Design review of the part built by this model. Coordinates are the model's own, in mm. A direction names the side the tool comes from. Coordinates: 2 decimals unless noted, no trailing zeros. Loops run counter-clockwise (first coordinate to the right, second up) from the corner with the lowest first, then second, coordinate; pieces in that order, holes last. Notation, with made-up numbers: (-39, 26) -> (-9, 26) arc R30 ccw to (-9, 52) -> close; hole circle Ø10 at (-24.5, -27). An arc over 180 degrees is marked (long way). Answer in a Markdown table with one row per item.
```python
from build123d import *

# Parameters (mm, degrees)
SKETCH3_R           = 2.4
BOSS_EXTRUDE1_DEPTH = 20
BOSS_EXTRUDE2_START = -15
SKETCH3_4_W         = 6.6
SKETCH3_4_H         = 6.6
SKETCH3_4_R         = 2.4
BOSS_EXTRUDE2_DEPTH = 15
BOSS_EXTRUDE3_DEPTH = 2


with BuildPart() as part:
    # Sketch3 → Boss-Extrude1 (new body)
    with BuildSketch(Plane.XY):
        Circle(SKETCH3_R)
    extrude(amount=BOSS_EXTRUDE1_DEPTH)

    # Sketch3_4 → Boss-Extrude2 (add)
    # profile 1 of 2: a face of its own
    with BuildSketch(Plane.XY.offset(BOSS_EXTRUDE2_START)):
        Rectangle(SKETCH3_4_W, SKETCH3_4_H)
        Circle(SKETCH3_4_R, mode=Mode.SUBTRACT)
    # profile 2 of 2: a face of its own
    with BuildSketch(Plane.XY.offset(BOSS_EXTRUDE2_START)):
        Circle(SKETCH3_4_R)
    extrude(amount=BOSS_EXTRUDE2_DEPTH)

    # Sketch3_5 → Boss-Extrude3 (add)
    with BuildSketch(Plane.XY):
        Polygon((3.3, 3.3), (3.3, -3.3), (5.3, -3.3), (5.3, 5.3), (-5.3, 5.3), (-5.3, -3.3), (-3.3, -3.3), (-3.3, 3.3), align=None)
    extrude(amount=-BOSS_EXTRUDE3_DEPTH)


solid = part.part
```
(1) To check wall thickness, follow probe 1 along X at (y, z) = (1, -13); probe 2 along Z at (x, y) = (2, 3); probe 3 along Z at (x, y) = (4.25, 4). State the ranges of each line that lie inside material, in increasing order.
Evaluation:
| item | result |
|---|---|
| probe 1 | x = -3.3 to 3.3 |
| probe 2 | z = -15 to 0 |
| probe 3 | z = -2 to 0 |
(2) Take a section at A-A on x = 0. Give the boundary of the cut face in (y, z), and give its area (3 significant figures).
Evaluation:
| item | result |
|---|---|
| outline | (-3.3, -15) -> (3.3, -15) -> (3.3, -2) -> (5.3, -2) -> (5.3, 0) -> (2.4, 0) -> (2.4, 20) -> (-2.4, 20) -> (-2.4, 0) -> (-3.3, 0) -> close |
| area | 199 mm² |
(3) For pin 1 (2 mm diameter, centred on x = 3.5, z = 2, fed in from +Y); pin 2 (2 mm diameter, centred on y = -1.5, z = -9, fed in from +X); pin 3 (3 mm diameter, centred on y = -2, z = 2, fed in from -X); pin 4 (5.5 mm diameter, centred on x = 1, z = -9.5, fed in from +Y), all flat-tipped, find the tip position at first contact; note any pin that passes through.
Evaluation:
| item | result |
|---|---|
| pin 1 | passes through |
| pin 2 | stops at x = 3.3 |
| pin 3 | stops at x = -2.35 |
| pin 4 | stops at y = 3.3 |
(4) Take a section at C-C on z = -11.5. Give the boundary of the cut face in (x, y), and give its area (3 significant figures).
Evaluation:
| item | result |
|---|---|
| outline | (-3.3, -3.3) -> (3.3, -3.3) -> (3.3, 3.3) -> (-3.3, 3.3) -> close |
| area | 43.6 mm² |
(5) Take a section at D-D on y = -1.5. Give the boundary of the cut face in (x, z), and give its area (3 significant figures).
Evaluation:
| item | result |
|---|---|
| outline | (-5.3, -2) -> (-3.3, -2) -> (-3.3, -15) -> (3.3, -15) -> (3.3, -2) -> (5.3, -2) -> (5.3, 0) -> (1.87, 0) -> (1.87, 20) -> (-1.87, 20) -> (-1.87, 0) -> (-5.3, 0) -> close |
| area | 182 mm² |
(6) Take a section at B-B on y = 0. Give the boundary of the cut face in (x, z).
Evaluation:
| item | result |
|---|---|
| outline | (-5.3, -2) -> (-3.3, -2) -> (-3.3, -15) -> (3.3, -15) -> (3.3, -2) -> (5.3, -2) -> (5.3, 0) -> (2.4, 0) -> (2.4, 20) -> (-2.4, 20) -> (-2.4, 0) -> (-5.3, 0) -> close |
(7) Tool access review of faces 1 (the flat face through (0, 3.3, -9)), 2 (the flat face through (3.3, 0, -9)), 3 (the cylindrical face through (1.29, 2.024, 9.86)), 4 (the flat face through (-3.3, 0, -9)), 5 (the flat face through (0, 5.3, -1)): name each direction out of +Z, -Z, +X, -X, +Y, -Y from which nothing blocks a thin tool from reaching the whole face with its end or side.
Evaluation:
| item | result |
|---|---|
| face 1 | -Z, +X, -X, +Y |
| face 2 | -Z, +X, +Y, -Y |
| face 3 | +Z |
| face 4 | -Z, -X, +Y, -Y |
| face 5 | +Z, -Z, +X, -X, +Y |
